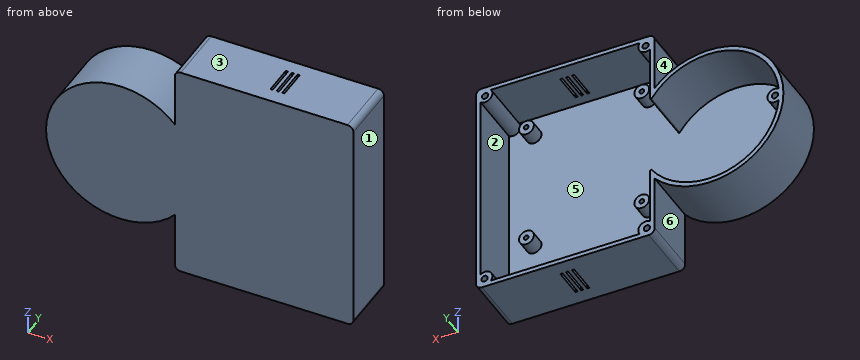
```python
from build123d import *

# Parameters (mm, degrees)
SKETCH8_W                      = 120
SKETCH8_H                      = 150
BOSS_EXTRUDE3_DEPTH            = 40
SKETCH9_R                      = 50
BOSS_EXTRUDE4_DEPTH            = 40
SHELL1_START                   = 3
SHELL1_DEPTH                   = 37
FILLET2_R                      = 0.5
SKETCH17_R                     = 5
BOSS_EXTRUDE6_DEPTH            = 10
CUT_EXTRUDE9_DEPTH             = 203.818558951
CUT_EXTRUDE9_DEPTH_BACK        = 203.818558951
SKETCH11_W                     = 1.5
SKETCH11_H                     = 20
CUT_EXTRUDE10_DEPTH            = 205.88547515
CUT_EXTRUDE10_DEPTH_BACK       = 205.88547515
SKETCH12_W                     = 1.5
SKETCH12_H                     = 20
CUT_EXTRUDE11_DEPTH            = 203.818558951
CUT_EXTRUDE11_DEPTH_BACK       = 203.818558951
SKETCH15_W                     = 1.5
SKETCH15_H                     = 20
SKETCH28_R                     = 5
BOSS_EXTRUDE7_DEPTH            = 37
SKETCH29_R                     = 5
BOSS_EXTRUDE8_DEPTH            = 40
SKETCH30_R                     = 5
BOSS_EXTRUDE9_DEPTH            = 40
SKETCH31_R                     = 5
BOSS_EXTRUDE10_DEPTH           = 37
SKETCH32_R                     = 5
BOSS_EXTRUDE11_DEPTH           = 37
F_2_0_221_DIAMETER_HOLE1_D     = 4.25
F_2_0_221_DIAMETER_HOLE1_DEPTH = 8
F_2_0_221_DIAMETER_HOLE1_TIP   = 1.276828815
F_2_0_221_DIAMETER_HOLE2_D     = 3.2
F_2_0_221_DIAMETER_HOLE2_DEPTH = 6
F_2_0_221_DIAMETER_HOLE2_TIP   = 0.96137699
FILLET3_R                      = 4


# Read off the part's stored shape, not the designer's step: Shell1
with BuildPart() as part:
    # Sketch8 → Boss-Extrude3 (new body)
    with BuildSketch(Plane(origin=(0, 0, 0), x_dir=(1, 0, 0), z_dir=(0, 1, 0))):
        with Locations((73.708855083, 72.164227744)):
            Rectangle(SKETCH8_W, SKETCH8_H)
    extrude(amount=BOSS_EXTRUDE3_DEPTH)

    # Sketch9 → Boss-Extrude4 (add)
    with BuildSketch(Plane(origin=(0, 0, 0), x_dir=(1, 0, 0), z_dir=(0, 1, 0))):
        with Locations((-22.779007595, 71.748458752)):
            Circle(SKETCH9_R)
    extrude(amount=BOSS_EXTRUDE4_DEPTH)

    # Shell1 outline → Shell1 (cut)
    with BuildSketch(Plane(origin=(0, 0, 0), x_dir=(1, 0, 0), z_dir=(0, 1, 0)).offset(SHELL1_START)):
        with BuildLine():
            Line((16.708855083, 46.259074664), (16.708855083, 0.164227744))
            Line((16.708855083, 0.164227744), (130.708855083, 0.164227744))
            Line((130.708855083, 0.164227744), (130.708855083, 144.164227744))
            Line((130.708855083, 144.164227744), (16.708855083, 144.164227744))
            Line((16.708855083, 144.164227744), (16.708855083, 97.237842839))
            ThreePointArc((16.708855083, 97.237842839), (-69.779007595, 71.748458751), (16.708855083, 46.259074664))
        make_face()
    extrude(amount=SHELL1_DEPTH, mode=Mode.SUBTRACT)

    # Fillet2
    fillet2_edges = [part.edges().sort_by_distance(p)[0] for p in [
        (16.708855083, 21.5, -46.259074664),
        (16.708855083, 21.5, -97.237842839),
    ]]
    fillet(fillet2_edges, radius=FILLET2_R)

    # Sketch17 → Boss-Extrude6 (add)
    with BuildSketch(Plane(origin=(1.848761015, 3, -2.465014687), x_dir=(1, 0, 0), z_dir=(0, 1, 0))):
        with Locations(Location((111.867013496, 11.175325825, 0), (0, 0, 270))):
            Circle(SKETCH17_R)
        with Locations(Location((34.367013496, 11.175325825, 0), (0, 0, 270))):
            Circle(SKETCH17_R)
        with Locations(Location((111.867013496, 94.175325825, 0), (0, 0, 270))):
            Circle(SKETCH17_R)
        with Locations(Location((34.367013496, 94.175325825, 0), (0, 0, 270))):
            Circle(SKETCH17_R)
    extrude(amount=BOSS_EXTRUDE6_DEPTH)

    # Sketch11 → Cut-Extrude9 (cut, two sides: drawn at the far end of the back side and taken through both)
    with BuildSketch(Plane.XY.offset(-CUT_EXTRUDE9_DEPTH_BACK)):
        with Locations((73.491480368, 20.290686907)):
            Rectangle(SKETCH11_W, SKETCH11_H)
    extrude(amount=CUT_EXTRUDE9_DEPTH + CUT_EXTRUDE9_DEPTH_BACK, mode=Mode.SUBTRACT)

    # Sketch12 → Cut-Extrude10 (cut, two sides: drawn at the far end of the back side and taken through both)
    with BuildSketch(Plane.XY.offset(2.835772256).offset(-CUT_EXTRUDE10_DEPTH_BACK)):
        with Locations((77.588922832, 20.290686907)):
            Rectangle(SKETCH12_W, SKETCH12_H)
    extrude(amount=CUT_EXTRUDE10_DEPTH + CUT_EXTRUDE10_DEPTH_BACK, mode=Mode.SUBTRACT)

    # Sketch15 → Cut-Extrude11 (cut, two sides: drawn at the far end of the back side and taken through both)
    with BuildSketch(Plane.XY.offset(-CUT_EXTRUDE11_DEPTH_BACK)):
        with Locations((81.379057112, 20.290686907)):
            Rectangle(SKETCH15_W, SKETCH15_H)
    extrude(amount=CUT_EXTRUDE11_DEPTH + CUT_EXTRUDE11_DEPTH_BACK, mode=Mode.SUBTRACT)

    # Sketch28 → Boss-Extrude7 (add)
    with BuildSketch(Plane(origin=(0, 3, 0), x_dir=(1, 0, 0), z_dir=(0, 1, 0))):
        with Locations((19.708855083, 141.164227744)):
            Circle(SKETCH28_R)
    extrude(amount=BOSS_EXTRUDE7_DEPTH)

    # Sketch29 → Boss-Extrude8 (add)
    with BuildSketch(Plane(origin=(0, 0, 0), x_dir=(1, 0, 0), z_dir=(0, 1, 0))):
        with Locations((19.708855083, 3.164227744)):
            Circle(SKETCH29_R)
    extrude(amount=BOSS_EXTRUDE8_DEPTH)

    # Sketch30 → Boss-Extrude9 (add)
    with BuildSketch(Plane(origin=(0, 0, 0), x_dir=(1, 0, 0), z_dir=(0, 1, 0))):
        with Locations((127.708855083, 141.164227744)):
            Circle(SKETCH30_R)
    extrude(amount=BOSS_EXTRUDE9_DEPTH)

    # Sketch31 → Boss-Extrude10 (add)
    with BuildSketch(Plane(origin=(0, 3, 0), x_dir=(1, 0, 0), z_dir=(0, 1, 0))):
        with Locations((127.708855083, 3.164227744)):
            Circle(SKETCH31_R)
    extrude(amount=BOSS_EXTRUDE10_DEPTH)

    # Sketch32 → Boss-Extrude11 (add)
    with BuildSketch(Plane(origin=(0, 3, 0), x_dir=(1, 0, 0), z_dir=(0, 1, 0))):
        with Locations((-67.018543515, 71.628998297)):
            Circle(SKETCH32_R)
    extrude(amount=BOSS_EXTRUDE11_DEPTH)

    # #2 (0.221) Diameter Hole1
    with Locations(Plane(origin=(0, 40, 0), x_dir=(1, 0, 0), z_dir=(0, 1, 0))):
        with Locations((18.917123201, 141.531370062), (127.969984407, 141.269223761), (127.602547564, 3.45328248), (19.774147178, 3.570575466), (-67.115618064, 71.668740496)):
            Hole(F_2_0_221_DIAMETER_HOLE1_D / 2, depth=F_2_0_221_DIAMETER_HOLE1_DEPTH)
            with Locations((0, 0, -(F_2_0_221_DIAMETER_HOLE1_DEPTH + F_2_0_221_DIAMETER_HOLE1_TIP / 2))):  # 118° drill point
                Cone(0, F_2_0_221_DIAMETER_HOLE1_D / 2, F_2_0_221_DIAMETER_HOLE1_TIP, mode=Mode.SUBTRACT)

    # #2 (0.221) Diameter Hole2
    with Locations(Plane(origin=(0, 13, 0), x_dir=(1, 0, 0), z_dir=(0, 1, 0))):
        with Locations((113.866576204, 96.665654076), (36.269140625, 13.672370328), (113.866576204, 13.415425177), (36.224664422, 96.637257854)):
            Hole(F_2_0_221_DIAMETER_HOLE2_D / 2, depth=F_2_0_221_DIAMETER_HOLE2_DEPTH)
            with Locations((0, 0, -(F_2_0_221_DIAMETER_HOLE2_DEPTH + F_2_0_221_DIAMETER_HOLE2_TIP / 2))):  # 118° drill point
                Cone(0, F_2_0_221_DIAMETER_HOLE2_D / 2, F_2_0_221_DIAMETER_HOLE2_TIP, mode=Mode.SUBTRACT)

    # Fillet3
    fillet3_edges = [part.edges().sort_by_distance(p)[0] for p in [
        (13.708855083, 20, -147.164227744),
        (133.708855083, 20, -147.164227744),
        (133.708855083, 20, 2.835772256),
        (13.708855083, 20, 2.835772256),
    ]]
    fillet(fillet3_edges, radius=FILLET3_R)


solid = part.part
```
Verification items for the finished model (mm, model axes). Face numbers are marked on the shaded views. A direction names the side the tool comes from. Coordinates: 2 decimals unless noted, no trailing zeros. Write each loop counter-clockwise with the first axis right and the second up, starting at its lowest first coordinate (ties: lowest second). Pieces come first, ordered by that corner, then holes. Notation, with made-up numbers: M 17,63 L 24,63 A22 cw 24,69 Z; hole C 32.5,19.5 d7. An arc over 180 degrees is marked long. Answer as a JSON object with one key per item and string values. Group by question number.
(1) Material ranges on line 1 (Z direction, x = 52, y = 28.5); line 2 (X direction, y = 32, z = -18.5); line 3 (X direction, y = 3.5, z = -39.5), recorded low to high.
(2) Cross-section at A-A, the plane z = -32.5. Record the cut outline in (x, y), and give its area (3 significant figures).
(3) Cross-section at C-C, the plane y = 36. State how many separate pieces and enclosed holes the cut face has, and give its area (3 significant figures).
(4) Release check for a two-part mould opening along X. For the marked faces 1, 2 and 3 record: +X half, -X half, draft (parallel to the pull), parting line (faces both ways), or undercut.
(5) Cross-section at B-B, the plane x = 93. Record the cut outline in (y, z).
(6) Tool access check on the marked faces 4, 5 and 6. Record the directions out of +Z, -Z, +X, -X, +Y, -Y that give a thin tool (end or side, any length) a straight path to the whole face; none if there is none.
(7) Cross-section at D-D, the plane z = -60. Record the cut outline in (x, y), and give its area (3 significant figures).
(8) Gauge pin test, flat ends, axial feed: pin 1 (3 mm diameter, centred on x = 36.22, z = -96.64, fed in from +Y); pin 2 (10 mm diameter, centred on x = -46, y = 21, fed in from -Z); pin 3 (6 mm diameter, centred on x = -40, y = 11, fed in from -Z). Record the tip position at first contact, or that the pin passes through.
Reply:
{
 "1": {"line 1": "-147.16 to -144.16, -0.16 to 2.84", "line 2": "13.71 to 16.71, 130.71 to 133.71", "line 3": "-60.99 to -56.97, 11.41 to 16.71, 130.71 to 133.71"},
 "2": {"outline": "M -53.76,0 L 8.2,0 L 8.2,40 L 3.08,40 L 3.08,3 L -48.64,3 L -48.64,40 L -53.76,40 Z; M 13.71,0 L 133.71,0 L 133.71,40 L 130.71,40 L 130.71,3 L 16.71,3 L 16.71,40 L 13.71,40 Z", "area": "1,150 mm²"},
 "3": {"separate pieces": "1", "enclosed holes": "6", "area": "2,330 mm²"},
 "4": {"face 1": "+X half", "face 2": "undercut", "face 3": "draft"},
 "5": {"outline": "M 0,-147.16 L 40,-147.16 L 40,-144.16 L 3,-144.16 L 3,-0.16 L 40,-0.16 L 40,2.84 L 0,2.84 Z"},
 "6": {"face 4": "+Z, +Y, -Y", "face 5": "+Y", "face 6": "-Z, +Y, -Y"},
 "7": {"outline": "M -71.38,0 L 133.71,0 L 133.71,40 L 130.71,40 L 130.71,3 L -68.29,3 L -68.29,40 L -71.38,40 Z", "area": "841 mm²"},
 "8": {"pin 1": "y = 6.94", "pin 2": "z = -118.31", "pin 3": "z = -119.68"}
}
